Drawing for the job (mm, zero at the part's lowest x, y, z). Give positions to 0.01 mm unless a question says otherwise; leave off trailing zeros. Order: outer loops, then holes, each group sorted by start corner. A loop starts at its lowest first (then second) coordinate and runs counter-clockwise, first axis right, second up. Notation, with made-up numbers: (-25.75, 65.5) -> (24.25, 65.5) arc R8 cw to (24.25, 80.5) -> close; hole circle Ø11 at (-5.5, -38). An arc over 180 degrees is marked (long way). Use one line per item in the form item = value. Start each with the question number.
1) Cut at C-C, the plane y = 0.5. Give the cut face in (x, z), and give its area (3 significant figures).
2) Cut at A-A, the plane z = 32.5. Give the cut face in (x, y).
3) Drop a flat-ended pin along its axis: P1, Ø12, axis at x = 98, z = 33, coming from the -Y side. Give the stop position or say it passes through.
4) Cut at B-B, the plane x = 56. Give the cut face in (y, z), and give its area (3 significant figures).
5) Cut at D-D, the plane x = 32.5. Give the cut face in (y, z), and give its area (3 significant figures).
6) Probe line 1 (Z direction, x = 95, y = 2.75); line 2 (X direction, y = 1.75, z = 9); line 3 (X direction, y = 0.8, z = 32.5). List the from-to ranges inside material, lowest first.
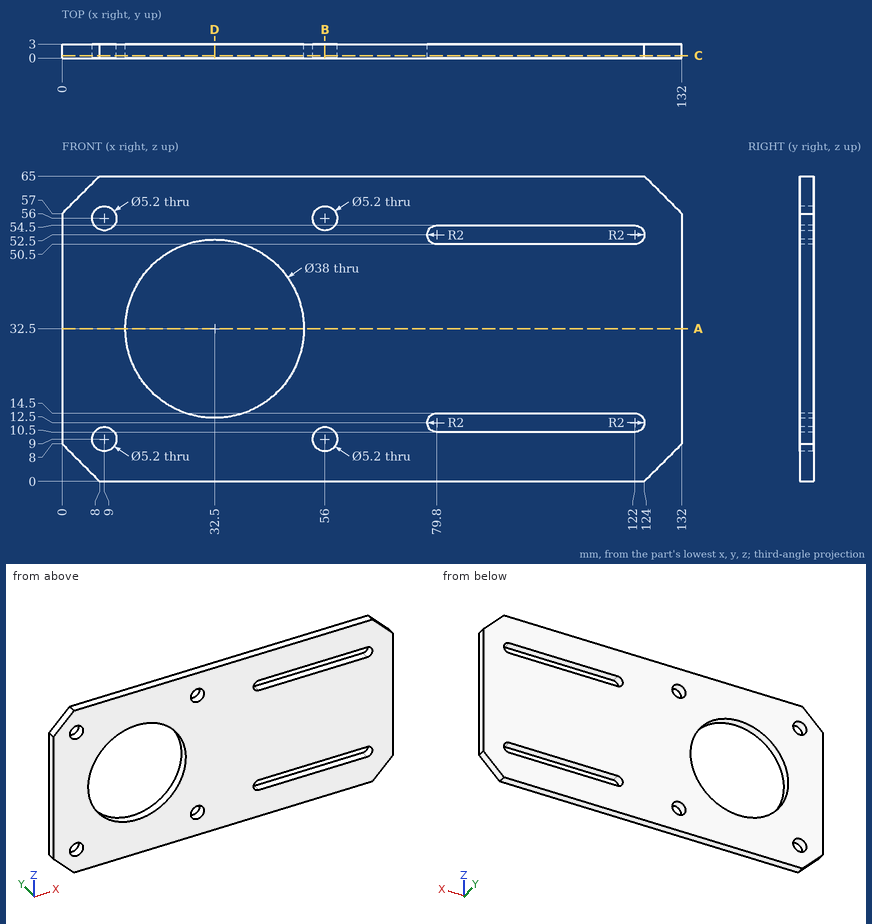
Result:
q1.outline = (0, 8) -> (8, 0) -> (124, 0) -> (132, 8) -> (132, 57) -> (124, 65) -> (8, 65) -> (0, 57) -> close; hole circle Ø5.2 at (9, 9); hole circle Ø5.2 at (9, 56); hole circle Ø38 at (32.5, 32.5); hole circle Ø5.2 at (56, 9); hole circle Ø5.2 at (56, 56); hole (79.8, 10.5) -> (122, 10.5) arc R2 ccw to (122, 14.5) -> (79.8, 14.5) arc R2 ccw to start; hole (79.8, 50.5) -> (122, 50.5) arc R2 ccw to (122, 54.5) -> (79.8, 54.5) arc R2 ccw to start
q1.area = 6,870 mm²
q2.outline = (0, 0) -> (13.5, 0) -> (13.5, 3) -> (0, 3) -> close; (51.5, 0) -> (132, 0) -> (132, 3) -> (51.5, 3) -> close
q3.P1 = 0
q4.outline = (0, 0) -> (3, 0) -> (3, 6.4) -> (0, 6.4) -> close; (0, 11.6) -> (3, 11.6) -> (3, 53.4) -> (0, 53.4) -> close; (0, 58.6) -> (3, 58.6) -> (3, 65) -> (0, 65) -> close
q4.area = 164 mm²
q5.outline = (0, 0) -> (3, 0) -> (3, 13.5) -> (0, 13.5) -> close; (0, 51.5) -> (3, 51.5) -> (3, 65) -> (0, 65) -> close
q5.area = 81.0 mm²
q6.line_1 = 0 to 10.5, 14.5 to 50.5, 54.5 to 65
q6.line_2 = 0 to 6.4, 11.6 to 53.4, 58.6 to 132
q6.line_3 = 0 to 13.5, 51.5 to 132
